Geometry: final body of the model. Coordinates: model frame, mm. Face numbers are marked on the shaded views. A direction names the side the tool comes from. Coordinates: 2 decimals unless noted, no trailing zeros. Loops run counter-clockwise (first coordinate to the right, second up) from the corner with the lowest first, then second, coordinate; pieces in that order, holes last. Notation, with made-up numbers: (37.5, 50.25) -> (82.5, 50.25) arc R17 cw to (82.5, 81.25) -> close; hole circle Ø3 at (-24, 20). An arc over 180 degrees is marked (long way). One line per item, written item: value. Start each with the question number.
Item 1: Section query B-B on z = 5.5. Return loops of the section in (x, y), then the cut area to 3 significant figures.
Item 2: Ray query, probe 1 along Y at (x, z) = (255, 12.5); probe 2 along Y at (x, z) = (257, 14.75); probe 3 along X at (y, z) = (-16.5, 17.25). Return the intervals inside material, ascending. Write a range as from..to.
Item 3: Contact query for flat-ended pins moving along their axis: pin 1 Ø6.5 at (x, z) = (236, 4) entering from +Y; pin 2 Ø8 at (x, y) = (255, 64) entering from +Z; pin 3 Ø5 at (x, y) = (238.5, 64) entering from -Z. Output: stop coordinate, or through.
Item 4: Section query C-C on z = 11.5. Return loops of the section in (x, y), then the cut area to 3 significant figures.
Item 5: Section query D-D on x = 255. Give the number of separate pieces and of enclosed holes in the cut face, then the cut area to 3 significant figures.
Item 6: Section query A-A on y = 39. Return loops of the section in (x, z), then the cut area to 3 significant figures.
Item 7: Mould query, pull axis X, two halves, no side actions, for the marked faces 1, 2 and 3. Classes: +X half, -X half, draft (parallel to the pull), parting line (faces both ways), or undercut.
Item 8: Set-up query: the marked faces 4, 5, 6 and 7. Return all of +Z, -Z, +X, -X, +Y, -Y with unobstructed straight access to the full face (end or side cutting, diameter ignored); none if empty.
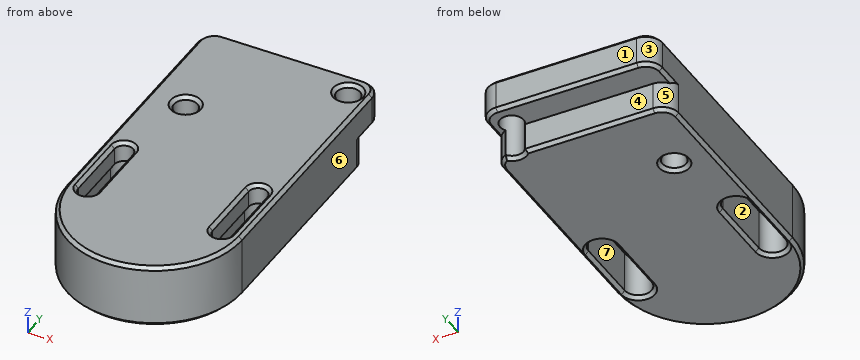
from build123d import *

# Parameters (mm, degrees)
SKETCH1_R           = 3.5
BOSS_EXTRUDE1_DEPTH = 19
CUT_EXTRUDE1_DEPTH  = 272.151249306
CUT_EXTRUDE2_DEPTH  = 272.151249306
CUT_EXTRUDE3_DEPTH  = 13
SKETCH5_W           = 9
SKETCH5_H           = 9
CUT_EXTRUDE4_DEPTH  = 91.033327163
FILLET1_R           = 5
CHAMFER1_SIZE       = 1


# Some blends are built 0.0001 mm under size
with BuildPart() as part:
    # Sketch1 → Boss-Extrude1 (new body)
    with BuildSketch(Plane.XY):
        Polygon((261, 71), (260, 71), (255, 71), (210, 71), (209, 71), (209, 41), (209, -59), (210, -59), (260, -59), (261, -59), align=None)
        with Locations((255, 64)):
            Circle(SKETCH1_R, mode=Mode.SUBTRACT)
        with Locations((220, 39)):
            Circle(SKETCH1_R, mode=Mode.SUBTRACT)
    extrude(amount=BOSS_EXTRUDE1_DEPTH)

    # Sketch2 → Cut-Extrude1 (cut, through all)
    with BuildSketch(Plane.XY.offset(19)):
        with BuildLine():
            Line((209, -59), (261, -59))
            Line((261, -59), (261, -6))
            ThreePointArc((261, -6), (235, -32), (209, -6))
            Line((209, -6), (209, -59))
        make_face()
    extrude(amount=-CUT_EXTRUDE1_DEPTH, mode=Mode.SUBTRACT)

    # Sketch3 → Cut-Extrude2 (cut, through all)
    with BuildSketch(Plane.XY.offset(19)):
        with BuildLine():
            Line((212.225, 14), (212.225, -6))
            ThreePointArc((212.225, -6), (215, -8.775), (217.775, -6))
            Line((217.775, -6), (217.775, 14))
            ThreePointArc((217.775, 14), (215, 16.775), (212.225, 14))
        make_face()
        with BuildLine():
            Line((252.225, 14), (252.225, -6))
            ThreePointArc((252.225, -6), (255, -8.775), (257.775, -6))
            Line((257.775, -6), (257.775, 14))
            ThreePointArc((257.775, 14), (255, 16.775), (252.225, 14))
        make_face()
    extrude(amount=-CUT_EXTRUDE2_DEPTH, mode=Mode.SUBTRACT)

    # Sketch4 → Cut-Extrude3 (cut)
    with BuildSketch(Plane(origin=(0, 0, 0), x_dir=(-1, 0, 0), z_dir=(0, 0, -1))):
        with BuildLine():
            Line((-251, 14), (-251, -6))
            ThreePointArc((-251, -6), (-255, -10), (-259, -6))
            Line((-259, -6), (-259, 14))
            ThreePointArc((-259, 14), (-255, 18), (-251, 14))
        make_face()
        with BuildLine():
            Line((-219, 14), (-219, -6))
            ThreePointArc((-219, -6), (-215, -10), (-211, -6))
            Line((-211, -6), (-211, 14))
            ThreePointArc((-211, 14), (-215, 18), (-219, 14))
        make_face()
    extrude(amount=-CUT_EXTRUDE3_DEPTH, mode=Mode.SUBTRACT)

    # Sketch5 → Cut-Extrude4 (cut, through all)
    with BuildSketch(Plane(origin=(261, 0, 0), x_dir=(0, 0, -1), z_dir=(1, 0, 0))):
        with Locations((-4.5, 66.5)):
            Rectangle(SKETCH5_W, SKETCH5_H)
    extrude(amount=-CUT_EXTRUDE4_DEPTH, mode=Mode.SUBTRACT)

    # Fillet1
    # the kernel refuses this fillet: 5 mm, written as the material it takes off along each edge
    with BuildSketch(Plane(origin=(209, 62, 9), x_dir=(0, -1, 0), z_dir=(0, 0, -1))) as fillet1_piece_1:
        with BuildLine():
            CenterArc((FILLET1_R, -FILLET1_R), FILLET1_R, 90, 90)
            Line((0, -FILLET1_R), (-FILLET1_R * 0.02, -FILLET1_R))
            Line((-FILLET1_R * 0.02, -FILLET1_R), (-FILLET1_R * 0.02, FILLET1_R * 0.02))
            Line((-FILLET1_R * 0.02, FILLET1_R * 0.02), (FILLET1_R, FILLET1_R * 0.02))
            Line((FILLET1_R, FILLET1_R * 0.02), (FILLET1_R, 0))
        make_face()
    extrude(amount=21.5, mode=Mode.SUBTRACT)
    with BuildSketch(Plane(origin=(261, 62, 9), x_dir=(0, -1, 0), z_dir=(0, 0, -1))) as fillet1_piece_2:
        with BuildLine():
            CenterArc((4.636222886, 5), FILLET1_R, 201.990710665, 68.009289335)
            Line((0, 3.127718677), (-0.092724458, 3.09027305))
            ThreePointArc((-0.092724458, 3.09027305), (-0.1, 1.563859338), (-0.1, 0))
            Line((-0.1, 0), (0, -0.1))
            Line((0, -0.1), (4.636222886, -0.1))
            Line((4.636222886, -0.1), (4.636222886, 0))
        make_face()
    extrude(amount=20.590557214, mode=Mode.SUBTRACT)
    with BuildSketch(Plane(origin=(209, 71, -3.5), x_dir=(1, 0, 0), z_dir=(0, 0, 1))) as fillet1_piece_3:
        with BuildLine():
            CenterArc((FILLET1_R, -FILLET1_R), FILLET1_R, 90, 90)
            Line((0, -FILLET1_R), (-FILLET1_R * 0.02, -FILLET1_R))
            Line((-FILLET1_R * 0.02, -FILLET1_R), (-FILLET1_R * 0.02, FILLET1_R * 0.02))
            Line((-FILLET1_R * 0.02, FILLET1_R * 0.02), (FILLET1_R, FILLET1_R * 0.02))
            Line((FILLET1_R, FILLET1_R * 0.02), (FILLET1_R, 0))
        make_face()
    extrude(amount=35, mode=Mode.SUBTRACT)
    with BuildSketch(Plane(origin=(261, 71, -3.5), x_dir=(-1, 0, 0), z_dir=(0, 0, 1))) as fillet1_piece_4:
        with BuildLine():
            CenterArc((FILLET1_R, FILLET1_R), FILLET1_R, 180, 90)
            Line((0, FILLET1_R), (-FILLET1_R * 0.02, FILLET1_R))
            Line((-FILLET1_R * 0.02, FILLET1_R), (-FILLET1_R * 0.02, -FILLET1_R * 0.02))
            Line((-FILLET1_R * 0.02, -FILLET1_R * 0.02), (FILLET1_R, -FILLET1_R * 0.02))
            Line((FILLET1_R, -FILLET1_R * 0.02), (FILLET1_R, 0))
        make_face()
    extrude(amount=35, mode=Mode.SUBTRACT)

    # Chamfer1
    chamfer1_edges = [part.edges().sort_by_distance(p)[0] for p in [
        (255, 60.5, 0),
        (216.5, 39, 0),
        (251.5, 64, 19),
        (209, 61.5, 9),
        (209, 25.5, 0),
        (209, 30, 19),
        (233.063859338, 62, 0),
        (261, 25.681888557, 0),
        (260.144961195, 60.160077651, 0),
        (210.464466094, 60.535533906, 0),
        (261, 61.681888557, 9),
        (261, 30, 19),
        (235, 71, 9),
        (259.535533906, 69.535533906, 9),
        (210.464466094, 69.535533906, 9),
        (235, 71, 19),
        (259.535533906, 69.535533906, 19),
        (210.464466094, 69.535533906, 19),
        (235, -32, 0),
        (235, -32, 19),
        (255, 16.775, 19),
        (252.225, 4, 19),
        (255, -8.775, 19),
        (257.775, 4, 19),
        (215, 16.775, 19),
        (212.225, 4, 19),
        (215, -8.775, 19),
        (217.775, 4, 19),
        (216.5, 39, 19),
        (255, 18, 0),
        (259, 4, 0),
        (255, -10, 0),
        (251, 4, 0),
        (215, 18, 0),
        (219, 4, 0),
        (215, -10, 0),
        (211, 4, 0),
    ]]
    chamfer(chamfer1_edges, length=CHAMFER1_SIZE - 0.0001)  # a hair under: the kernel refuses the full size


solid = part.part
Reply:
1. outline: (209, -6) arc R26 ccw to (261, -6) -> (261, 57.36) arc R5 ccw to (257.87, 62) arc R3.5 cw to (252.13, 62) -> (214, 62) arc R5 ccw to (209, 57) -> close; hole (211, -6) arc R4 ccw to (219, -6) -> (219, 14) arc R4 ccw to (211, 14) -> close; hole circle Ø7 at (220, 39); hole (251, -6) arc R4 ccw to (259, -6) -> (259, 14) arc R4 ccw to (251, 14) -> close
1. area: 4,120 mm²
2. probe 1: y = -22.61..-10, 18..60.5, 67.5..71
2. probe 2: y = -19.86..-7.92, 15.92..61.13, 66.87..70.9
2. probe 3: x = 211.21..258.79
3. pin 1: stops at y = 62
3. pin 2: stops at z = 18.5
3. pin 3: stops at z = 0.5
4. outline: (209, -6) arc R26 ccw to (261, -6) -> (261, 66) arc R5 ccw to (256, 71) -> (214, 71) arc R5 ccw to (209, 66) -> close; hole (211, -6) arc R4 ccw to (219, -6) -> (219, 14) arc R4 ccw to (211, 14) -> close; hole circle Ø7 at (220, 39); hole (251, -6) arc R4 ccw to (259, -6) -> (259, 14) arc R4 ccw to (251, 14) -> close; hole circle Ø7 at (255, 64)
4. area: 4,560 mm²
5. separate pieces: 3
5. enclosed holes: 0
5. area: 1,090 mm²
6. outline: (209, 1) -> (210, 0) -> (215.5, 0) -> (216.5, 1) -> (216.5, 18) -> (215.5, 19) -> (210, 19) -> (209, 18) -> close; (223.5, 1) -> (224.5, 0) -> (260, 0) -> (261, 1) -> (261, 18) -> (260, 19) -> (224.5, 19) -> (223.5, 18) -> close
6. area: 851 mm²
7. face 1: draft
7. face 2: undercut
7. face 3: -X half
8. face 4: -Z, +X, -X, +Y
8. face 5: -Z, -X, +Y
8. face 6: +Z, -Z, +X, +Y, -Y
8. face 7: -Z
